from build123d import *

# Parameters (mm, degrees)
SKETCH1_R           = 10.16
SKETCH1_R_2         = 4.550000044
SKETCH1_R_3         = 3.550000044
BOSS_EXTRUDE1_DEPTH = 3.175
SKETCH2_R           = 4.550000044
SKETCH2_R_2         = 3.550000044
CUT_EXTRUDE1_DEPTH  = 1.524


with BuildPart() as part:
    # Sketch1 → Boss-Extrude1 (new body)
    # profile 1 of 5: a face of its own
    with BuildSketch(Plane(origin=(0, 0, 0), x_dir=(1, 0, 0), z_dir=(0, 1, 0))):
        with Locations(Location((0, 0, 0), (0, 0, 270))):
            Circle(SKETCH1_R)
        with Locations((0, 4.953)):
            Circle(SKETCH1_R_2, mode=Mode.SUBTRACT)
        with Locations((0, -4.953)):
            Circle(SKETCH1_R_2, mode=Mode.SUBTRACT)
    # profile 2 of 5: a face of its own
    with BuildSketch(Plane(origin=(0, 0, 0), x_dir=(1, 0, 0), z_dir=(0, 1, 0))):
        with Locations((0, 4.953)):
            Circle(SKETCH1_R_2)
        with Locations((0, 4.953)):
            Circle(SKETCH1_R_3, mode=Mode.SUBTRACT)
    # profile 3 of 5: a face of its own
    with BuildSketch(Plane(origin=(0, 0, 0), x_dir=(1, 0, 0), z_dir=(0, 1, 0))):
        with Locations((0, 4.953)):
            Circle(SKETCH1_R_3)
    # profile 4 of 5: a face of its own
    with BuildSketch(Plane(origin=(0, 0, 0), x_dir=(1, 0, 0), z_dir=(0, 1, 0))):
        with Locations((0, -4.953)):
            Circle(SKETCH1_R_2)
        with Locations((0, -4.953)):
            Circle(SKETCH1_R_3, mode=Mode.SUBTRACT)
    # profile 5 of 5: a face of its own
    with BuildSketch(Plane(origin=(0, 0, 0), x_dir=(1, 0, 0), z_dir=(0, 1, 0))):
        with Locations((0, -4.953)):
            Circle(SKETCH1_R_3)
    extrude(amount=BOSS_EXTRUDE1_DEPTH)

    # Sketch2 → Cut-Extrude1 (cut)
    # profile 1 of 2: a face of its own
    with BuildSketch(Plane.XZ):
        with Locations(Location((0, -4.953, 0), (0, 0, 270))):
            Circle(SKETCH2_R)
        with Locations(Location((0, -4.953, 0), (0, 0, 270))):
            Circle(SKETCH2_R_2, mode=Mode.SUBTRACT)
    # profile 2 of 2: a face of its own
    with BuildSketch(Plane.XZ):
        with Locations(Location((0, 4.953, 0), (0, 0, 270))):
            Circle(SKETCH2_R)
        with Locations(Location((0, 4.953, 0), (0, 0, 270))):
            Circle(SKETCH2_R_2, mode=Mode.SUBTRACT)
    extrude(amount=-CUT_EXTRUDE1_DEPTH, mode=Mode.SUBTRACT)


solid = part.part
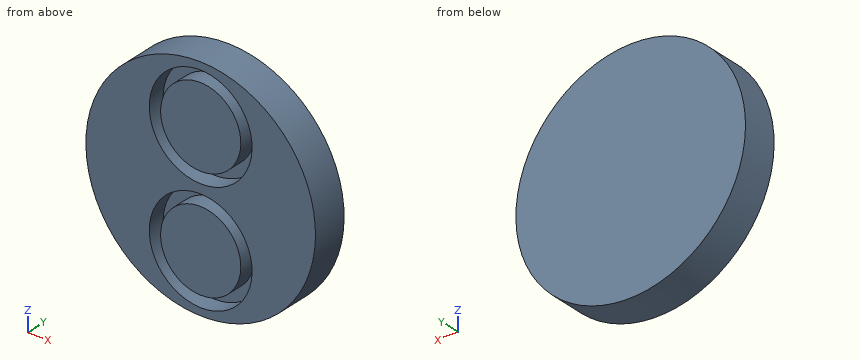
CAD build for the part. Positions are in the model's coordinates, mm. Round coordinates to 2 decimals unless told otherwise and drop trailing zeros. Loops run counter-clockwise (first coordinate to the right, second up) from the corner with the lowest first, then second, coordinate; pieces in that order, holes last. Notation, with made-up numbers: M 13,25.25 L 35,25.25 A23 cw 35,37.25 Z; hole C -1,-23.75 d2. An arc over 180 degrees is marked long. One line per question, with ' | ' between items. Start each with the question number.
Item 1: Cut at C-C, the plane x = 0. Write the cut outline in (y, z) (3 decimals).
Item 2: Cut at B-B, the plane z = 5.5. Write the cut outline in (x, y) (3 decimals).
Item 3: Cut at A-A, the plane y = 0.4. Write the cut outline in (x, z), plus the area to 3 significant figures.
Item 4: Cut at D-D, the plane y = 1.95. Write the cut outline in (x, z), plus the area to 3 significant figures.
Item 5: Wall check: line 1 (X direction, y = 0.65, z = 7); line 2 (X direction, y = 0.5, z = -7.5); line 3 (Z direction, x = 2.5, y = 0.4). Give the ranges that are in metal, low to high.
Item 6: Pin check, flat tip, straight feed: pin 1 Ø1 at (y, z) = (2.5, -7) entering from +X. Stop position of the tip, or through.
Responses:
1) outline: M 0,-10.16 L 3.175,-10.16 L 3.175,10.16 L 0,10.16 L 0,9.503 L 1.524,9.503 L 1.524,8.503 L 0,8.503 L 0,1.403 L 1.524,1.403 L 1.524,0.403 L 0,0.403 L 0,-0.403 L 1.524,-0.403 L 1.524,-1.403 L 0,-1.403 L 0,-8.503 L 1.524,-8.503 L 1.524,-9.503 L 0,-9.503 Z
2) outline: M -8.543,0 L -4.517,0 L -4.517,1.524 L -3.508,1.524 L -3.508,0 L 3.508,0 L 3.508,1.524 L 4.517,1.524 L 4.517,0 L 8.543,0 L 8.543,3.175 L -8.543,3.175 Z
3) outline: C 0,0 d20.32; C 0,-4.95 d7.1; C 0,4.95 d7.1; hole C 0,-4.95 d9.1; hole C 0,4.95 d9.1 | area: 273 mm²
4) outline: C 0,0 d20.32 | area: 324 mm²
5) line 1: x = -7.36 to -4.06, -2.9 to 2.9, 4.06 to 7.36 | line 2: x = -6.85 to -3.77, -2.47 to 2.47, 3.77 to 6.85 | line 3: z = -9.85 to -8.75, -7.47 to -2.43, -1.15 to 1.15, 2.43 to 7.47, 8.75 to 9.85
6) pin 1: stops at x = 7.81
